The listing builds one solid part. Answer for the finished solid, in the listing's coordinates (mm). A direction names the side the tool comes from. Round coordinates to 2 decimals unless told otherwise and drop trailing zeros. Write each loop counter-clockwise with the first axis right and the second up, starting at its lowest first coordinate (ties: lowest second). Pieces come first, ordered by that corner, then holes. Notation, with made-up numbers: M 75.25,-35 L 125.25,-35 A21 cw 125.25,-13 Z; hole C -17,40 d7. An arc over 180 degrees is marked long. Write each question's results on one line, items separated by ' | '.
from build123d import *

# Parameters (mm, degrees)
F0_R      = 43
F1_DEPTH  = 7.3
F2_R      = 38.3
F3_DEPTH  = 4.3
F4_R      = 43
F5_DEPTH  = 5.7
F6_R      = 38.3
F7_DEPTH  = 4.3
F8_R      = 43
F9_DEPTH  = 5.7
F10_R     = 38.3
F11_DEPTH = 4.3


with BuildPart() as f1:
    # F0 (on Top) → F1 (new body)
    with BuildSketch(Plane.XY):
        Circle(F0_R)
    extrude(amount=F1_DEPTH)

    # F2 (on face) → F3 (join)
    with BuildSketch(Plane(origin=(0, 0, 0), x_dir=(1, 0, 0), z_dir=(0, 0, -1))):
        Circle(F2_R)
    extrude(amount=F3_DEPTH)

    # F4 (on face) → F5 (join)
    with BuildSketch(Plane(origin=(0, 0, -4.3), x_dir=(1, 0, 0), z_dir=(0, 0, -1))):
        Circle(F4_R)
    extrude(amount=F5_DEPTH)

    # F6 (on face) → F7 (join)
    with BuildSketch(Plane(origin=(0, 0, -10), x_dir=(1, 0, 0), z_dir=(0, 0, -1))):
        Circle(F6_R)
    extrude(amount=F7_DEPTH)

    # F8 (on face) → F9 (join)
    with BuildSketch(Plane(origin=(0, 0, -14.3), x_dir=(1, 0, 0), z_dir=(0, 0, -1))):
        Circle(F8_R)
    extrude(amount=F9_DEPTH)

    # F10 (on face) → F11 (join)
    with BuildSketch(Plane(origin=(0, 0, -20), x_dir=(1, 0, 0), z_dir=(0, 0, -1))):
        Circle(F10_R)
    extrude(amount=F11_DEPTH)


solid = f1.part
1) Find the intervals of material crossed by line 1 (Z direction, x = 16, y = -37.5); line 2 (Y direction, x = -12.5, z = -5); line 3 (X direction, y = -31.5, z = 4.5), in increasing order.
Return value:
line 1: -20 to -14.3, -10 to -4.3, 0 to 7.3 | line 2: -41.14 to 41.14 | line 3: -29.27 to 29.27
2) The mould has two halves that part along Z. Classify faces 1 (the face through (-5.598, -42.634, -17.11)), 2 (the face through (-1, -1, -24.3)), 3 (the face through (-38.4, 3, -4.3)): +Z half, -Z half, draft (parallel to the pull), parting line (faces both ways), or undercut.
Return value:
face 1: draft | face 2: -Z half | face 3: undercut
3) Section C-C (z = -17.5) is taken. Determine the outline of the cut face in (x, y).
Return value:
outline: C 0,0 d86
4) A tool of negligible diameter and unlimited length cuts with its end or side. For faces 4 (the face through (-38.4, -3, 0)), 5 (the face through (-38.4, 3, -20)), 6 (the face through (-1, 1, 7.3)), from which of +Z, -Z, +X, -X, +Y, -Y can it reach the whole face along a straight path? Write none if from no direction.
Return value:
face 4: none | face 5: -Z | face 6: +Z, +X, -X, +Y, -Y
5) Section A-A (y = 0) is taken. Determine the outline of the cut face in (x, z).
Return value:
outline: M -43,-20 L -38.3,-20 L -38.3,-24.3 L 38.3,-24.3 L 38.3,-20 L 43,-20 L 43,-14.3 L 38.3,-14.3 L 38.3,-10 L 43,-10 L 43,-4.3 L 38.3,-4.3 L 38.3,0 L 43,0 L 43,7.3 L -43,7.3 L -43,0 L -38.3,0 L -38.3,-4.3 L -43,-4.3 L -43,-10 L -38.3,-10 L -38.3,-14.3 L -43,-14.3 Z
6) Each of these flat-tipped pins is pushed along its axis until it touches: pin 1 (6 mm diameter, centred on x = 19.5, z = 3.5, fed in from -Y); pin 2 (8 mm diameter, centred on x = -18.5, z = -3.5, fed in from +Y); pin 3 (10 mm diameter, centred on x = 19.5, z = -20, fed in from +Y). Where does it stop, or does it pass through?
Return value:
pin 1: y = -39.71 | pin 2: y = 40.45 | pin 3: y = 40.48
